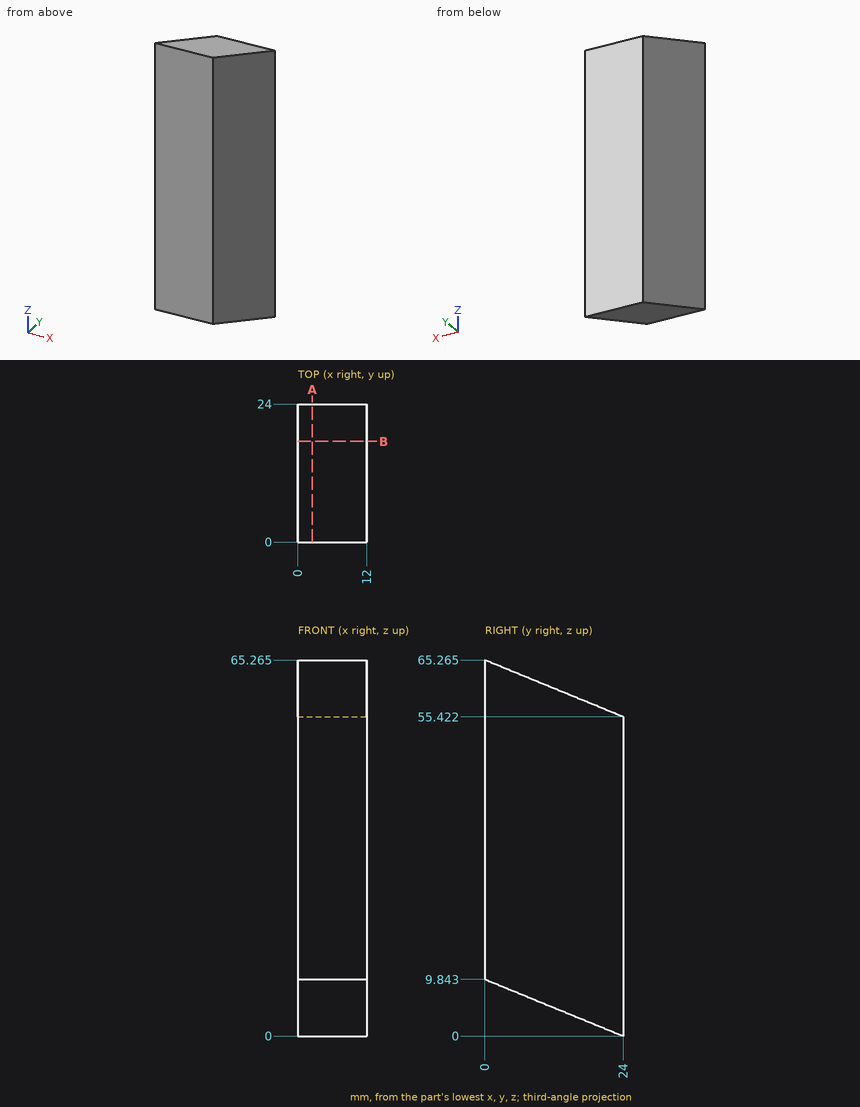
Answer from the drawing. Dimensions are ordinates in mm from the lowest x, y and z of the part. Coordinates: 2 decimals unless noted, no trailing zeros. Loops run counter-clockwise (first coordinate to the right, second up) from the corner with the lowest first, then second, coordinate; pieces in that order, holes last. Notation, with made-up numbers: (2, 17.5) - (27, 17.5) arc R18 ccw to (27, 22.5) - close; hole circle Ø4 at (-9.75, -6). An arc over 180 degrees is marked (long way). Answer in a Markdown table with one row per item.
1. Straight lines are drawn through the part: line 1 (Z direction, x = 7.75, y = 4.5); line 2 (Z direction, x = 3, y = 3.25); line 3 (Y direction, x = 2, z = 4.5). For each, find the intervals that lie inside material, in ascending order.
Conclusion:
| item | result |
|---|---|
| line 1 | z = 8 to 63.42 |
| line 2 | z = 8.51 to 63.93 |
| line 3 | y = 13.03 to 24 |
2. Given pin 1 (5 mm diameter, centred on x = 2, y = 11, fed in from +Z); pin 2 (2 mm diameter, centred on x = 9.5, y = 6.5, fed in from +Z); pin 3 (1.5 mm diameter, centred on x = 7, y = 10.5, fed in from -Z), each flat-ended and moving along its own axis, determine where each tip first touches the part or whether it passes through.
Conclusion:
| item | result |
|---|---|
| pin 1 | stops at z = 61.78 |
| pin 2 | stops at z = 63.01 |
| pin 3 | stops at z = 5.23 |
3. Find section A-A, the plane x = 2.5. Write down the section's boundary in (y, z) (3 decimals).
Conclusion:
| item | result |
|---|---|
| outline | (0, 9.843) - (24, 0) - (24, 55.422) - (0, 65.265) - close |
4. Find section B-B, the plane y = 17.5. Write down the section's boundary in (x, z), then the cut area to 3 significant figures.
Conclusion:
| item | result |
|---|---|
| outline | (0, 2.67) - (12, 2.67) - (12, 58.09) - (0, 58.09) - close |
| area | 665 mm² |
